Here's how the part is built. I have some questions about the finished solid (model axes, mm). Face numbers are marked on the shaded views. Coordinates: 2 decimals unless noted, no trailing zeros. Write each loop counter-clockwise with the first axis right and the second up, starting at its lowest first coordinate (ties: lowest second). Pieces come first, ordered by that corner, then holes. Notation, with made-up numbers: (30.25, 41.5) -> (38.25, 41.5) arc R16 cw to (38.25, 61.5) -> close; hole circle Ø8 at (-4, 62). An arc over 180 degrees is marked (long way). Put each result on its own line as item: value. Start each with the question number.
Item 1: I want a section at D-D, the plane y = 1.5. State how many separate pieces and enclosed holes the cut face has, then the cut area to 3 significant figures.
Item 2: I want a section at A-A, the plane x = -2.5. List the corners of the cut face in (y, z) for me, then the cut area to 3 significant figures.
Item 3: I want a section at B-B, the plane z = 2.5. List the corners of the cut face in (x, y) for me, then the cut area to 3 significant figures.
Item 4: I want a section at C-C, the plane x = -19.5. List the corners of the cut face in (y, z) for me, then the cut area to 3 significant figures.
Item 5: I need wall thicknesses on line 1 (X direction, y = 0.8, z = 15.66); line 2 (Z direction, x = 25.3, y = 0.75); line 3 (X direction, y = 1.45, z = -8.5). Which ranges of each line are inside material? Lowest first, please. Write a range as [from, to].
Item 6: If we mould it in two halves opening along Y, with no side actions, what happens to the marked faces 1 and 2? For each: released by +Y, released by -Y, zero draft, split by the parting line, or undercut.
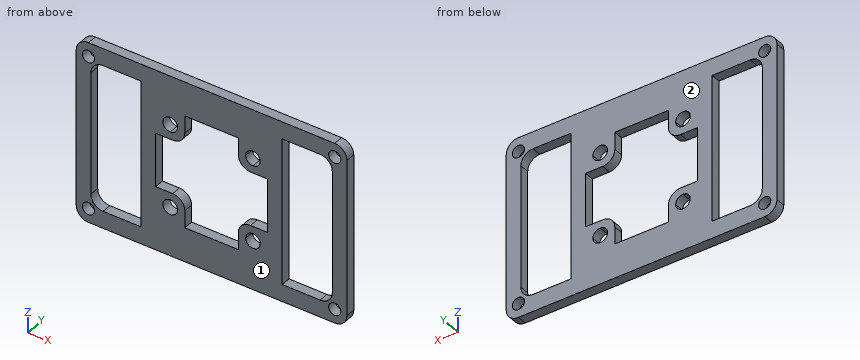
from build123d import *

# Parameters (mm, degrees)
SKETCH1_W           = 55.6
SKETCH1_H           = 37
BOSS_EXTRUDE1_DEPTH = 2
CUT_EXTRUDE2_REACH  = 4
FILLET2_R           = 2.5
CUT_EXTRUDE3_REACH  = 4
CUT_EXTRUDE4_REACH  = 4
SKETCH7_R           = 1.25
CUT_EXTRUDE5_DEPTH  = 10


with BuildPart() as part:
    # Sketch1 → Boss-Extrude1 (new body)
    with BuildSketch(Plane(origin=(0, 0, 0), x_dir=(1, 0, 0), z_dir=(0, 1, 0))):
        Rectangle(SKETCH1_W, SKETCH1_H)
    extrude(amount=BOSS_EXTRUDE1_DEPTH)

    # Sketch5 → Cut-Extrude2 (cut, up to next)
    with BuildSketch(Plane(origin=(0, 2, 0), x_dir=(1, 0, 0), z_dir=(0, 1, 0)), mode=Mode.PRIVATE) as cut_extrude2_sk1:
        with BuildLine():
            Line((5.5, 11.5), (-5.5, 11.5))
            Line((-5.5, 11.5), (-5.5, 8))
            ThreePointArc((-5.5, 8), (-6.232233047, 6.232233047), (-8, 5.5))
            Line((-8, 5.5), (-11.5, 5.5))
            Line((-11.5, 5.5), (-11.5, -5.5))
            Line((-11.5, -5.5), (-8, -5.5))
            ThreePointArc((-8, -5.5), (-6.232233047, -6.232233047), (-5.5, -8))
            Line((-5.5, -8), (-5.5, -11.5))
            Line((-5.5, -11.5), (5.5, -11.5))
            Line((5.5, -11.5), (5.5, -8))
            ThreePointArc((5.5, -8), (6.232233047, -6.232233047), (8, -5.5))
            Line((8, -5.5), (11.5, -5.5))
            Line((11.5, -5.5), (11.5, 5.5))
            Line((11.5, 5.5), (8, 5.5))
            ThreePointArc((8, 5.5), (6.232233047, 6.232233047), (5.5, 8))
            Line((5.5, 8), (5.5, 11.5))
        make_face()
    cut_extrude2_tool1 = extrude(cut_extrude2_sk1.sketch, amount=-CUT_EXTRUDE2_REACH, mode=Mode.PRIVATE) & part.part
    add(cut_extrude2_tool1.solids().sort_by_distance((0, 2, 0))[0], mode=Mode.SUBTRACT)

    # Fillet2
    fillet2_edges = [part.edges().sort_by_distance(p)[0] for p in [
        (27.8, 1, 18.5),
        (-27.8, 1, 18.5),
        (-27.8, 1, -18.5),
        (27.8, 1, -18.5),
    ]]
    fillet(fillet2_edges, radius=FILLET2_R)

    # Sketch6 → Cut-Extrude3 (cut, up to next)
    with BuildSketch(Plane(origin=(0, 2, 0), x_dir=(1, 0, 0), z_dir=(0, 1, 0)), mode=Mode.PRIVATE) as cut_extrude3_sk1:
        with BuildLine():
            Line((-22.3, 15), (-14.5, 15))
            Line((-14.5, 15), (-14.5, -15))
            Line((-14.5, -15), (-22.3, -15))
            ThreePointArc((-22.3, -15), (-24.067766953, -14.267766953), (-24.8, -12.5))
            Line((-24.8, -12.5), (-24.8, 12.5))
            ThreePointArc((-24.8, 12.5), (-24.067766953, 14.267766953), (-22.3, 15))
        make_face()
    cut_extrude3_tool1 = extrude(cut_extrude3_sk1.sketch, amount=-CUT_EXTRUDE3_REACH, mode=Mode.PRIVATE) & part.part
    add(cut_extrude3_tool1.solids().sort_by_distance((-19.60979, 2, 0))[0], mode=Mode.SUBTRACT)
    # Sketch6 → Cut-Extrude3 (cut, up to next)
    with BuildSketch(Plane(origin=(0, 2, 0), x_dir=(1, 0, 0), z_dir=(0, 1, 0)), mode=Mode.PRIVATE) as cut_extrude3_sk2:
        with BuildLine():
            Line((22.3, -15), (14.5, -15))
            Line((14.5, -15), (14.5, 15))
            Line((14.5, 15), (22.3, 15))
            ThreePointArc((22.3, 15), (24.067766953, 14.267766953), (24.8, 12.5))
            Line((24.8, 12.5), (24.8, -12.5))
            ThreePointArc((24.8, -12.5), (24.067766953, -14.267766953), (22.3, -15))
        make_face()
    cut_extrude3_tool2 = extrude(cut_extrude3_sk2.sketch, amount=-CUT_EXTRUDE3_REACH, mode=Mode.PRIVATE) & part.part
    add(cut_extrude3_tool2.solids().sort_by_distance((19.60979, 2, 0))[0], mode=Mode.SUBTRACT)

    # Sketch7 → Cut-Extrude4 (cut, up to next)
    with BuildSketch(Plane(origin=(0, 2, 0), x_dir=(1, 0, 0), z_dir=(0, 1, 0)), mode=Mode.PRIVATE) as cut_extrude4_sk1:
        with Locations((-25.3, 15.66)):
            Circle(SKETCH7_R)
    cut_extrude4_tool1 = extrude(cut_extrude4_sk1.sketch, amount=-CUT_EXTRUDE4_REACH, mode=Mode.PRIVATE) & part.part
    add(cut_extrude4_tool1.solids().sort_by_distance((-25.3, 2, -15.66))[0], mode=Mode.SUBTRACT)
    # Sketch7 → Cut-Extrude4 (cut, up to next)
    with BuildSketch(Plane(origin=(0, 2, 0), x_dir=(1, 0, 0), z_dir=(0, 1, 0)), mode=Mode.PRIVATE) as cut_extrude4_sk2:
        with Locations((25.3, 15.66)):
            Circle(SKETCH7_R)
    cut_extrude4_tool2 = extrude(cut_extrude4_sk2.sketch, amount=-CUT_EXTRUDE4_REACH, mode=Mode.PRIVATE) & part.part
    add(cut_extrude4_tool2.solids().sort_by_distance((25.3, 2, -15.66))[0], mode=Mode.SUBTRACT)
    # Sketch7 → Cut-Extrude4 (cut, up to next)
    with BuildSketch(Plane(origin=(0, 2, 0), x_dir=(1, 0, 0), z_dir=(0, 1, 0)), mode=Mode.PRIVATE) as cut_extrude4_sk3:
        with Locations((25.3, -15.66)):
            Circle(SKETCH7_R)
    cut_extrude4_tool3 = extrude(cut_extrude4_sk3.sketch, amount=-CUT_EXTRUDE4_REACH, mode=Mode.PRIVATE) & part.part
    add(cut_extrude4_tool3.solids().sort_by_distance((25.3, 2, 15.66))[0], mode=Mode.SUBTRACT)
    # Sketch7 → Cut-Extrude4 (cut, up to next)
    with BuildSketch(Plane(origin=(0, 2, 0), x_dir=(1, 0, 0), z_dir=(0, 1, 0)), mode=Mode.PRIVATE) as cut_extrude4_sk4:
        with Locations((-25.3, -15.66)):
            Circle(SKETCH7_R)
    cut_extrude4_tool4 = extrude(cut_extrude4_sk4.sketch, amount=-CUT_EXTRUDE4_REACH, mode=Mode.PRIVATE) & part.part
    add(cut_extrude4_tool4.solids().sort_by_distance((-25.3, 2, 15.66))[0], mode=Mode.SUBTRACT)

    # Sketch3 → Cut-Extrude5 (cut)
    with BuildSketch(Plane(origin=(0, 2, 0), x_dir=(1, 0, 0), z_dir=(0, 1, 0))):
        with BuildLine():
            Line((-8.5, 7), (-8.5, 8.5))
            Line((-8.5, 8.5), (-7, 8.5))
            ThreePointArc((-7, 8.5), (-9.560660172, 9.560660172), (-8.5, 7))
        make_face()
        with BuildLine():
            Line((-7, 8.5), (-8.5, 8.5))
            Line((-8.5, 8.5), (-8.5, 7))
            ThreePointArc((-8.5, 7), (-7.439339828, 7.439339828), (-7, 8.5))
        make_face()
        with BuildLine():
            ThreePointArc((10, 8.5), (8.5, 10), (7, 8.5))
            Line((7, 8.5), (8.5, 8.5))
            Line((8.5, 8.5), (8.5, 7))
            ThreePointArc((8.5, 7), (9.560660172, 7.439339828), (10, 8.5))
        make_face()
        with BuildLine():
            Line((8.5, 8.5), (7, 8.5))
            ThreePointArc((7, 8.5), (7.439339828, 7.439339828), (8.5, 7))
            Line((8.5, 7), (8.5, 8.5))
        make_face()
        with BuildLine():
            ThreePointArc((-7, -8.5), (-7.439339828, -7.439339828), (-8.5, -7))
            Line((-8.5, -7), (-8.5, -8.5))
            Line((-8.5, -8.5), (-7, -8.5))
        make_face()
        with BuildLine():
            Line((-8.5, -8.5), (-8.5, -7))
            ThreePointArc((-8.5, -7), (-9.560660172, -9.560660172), (-7, -8.5))
            Line((-7, -8.5), (-8.5, -8.5))
        make_face()
        with BuildLine():
            ThreePointArc((10, -8.5), (9.560660172, -7.439339828), (8.5, -7))
            Line((8.5, -7), (8.5, -8.5))
            Line((8.5, -8.5), (7, -8.5))
            ThreePointArc((7, -8.5), (8.5, -10), (10, -8.5))
        make_face()
        with BuildLine():
            Line((8.5, -8.5), (8.5, -7))
            ThreePointArc((8.5, -7), (7.439339828, -7.439339828), (7, -8.5))
            Line((7, -8.5), (8.5, -8.5))
        make_face()
    extrude(amount=-CUT_EXTRUDE5_DEPTH, mode=Mode.SUBTRACT)


solid = part.part
Calculated:
1. separate pieces: 1
1. enclosed holes: 11
1. area: 1,000 mm2
2. outline: (0, -18.5) -> (2, -18.5) -> (2, -11.5) -> (0, -11.5) -> close; (0, 11.5) -> (2, 11.5) -> (2, 18.5) -> (0, 18.5) -> close
2. area: 28.0 mm2
3. outline: (-27.8, 0) -> (-24.8, 0) -> (-24.8, 2) -> (-27.8, 2) -> close; (-14.5, 0) -> (-11.5, 0) -> (-11.5, 2) -> (-14.5, 2) -> close; (11.5, 0) -> (14.5, 0) -> (14.5, 2) -> (11.5, 2) -> close; (24.8, 0) -> (27.8, 0) -> (27.8, 2) -> (24.8, 2) -> close
3. area: 24.0 mm2
4. outline: (0, -18.5) -> (2, -18.5) -> (2, -15) -> (0, -15) -> close; (0, 15) -> (2, 15) -> (2, 18.5) -> (0, 18.5) -> close
4. area: 14.0 mm2
5. line 1: x = [-27.8, -26.55], [-24.05, 24.05], [26.55, 27.8]
5. line 2: z = [-18.5, -16.91], [-14.41, 14.41], [16.91, 18.5]
5. line 3: x = [-27.8, -24.8], [-14.5, -10], [-7, -5.5], [5.5, 7], [10, 14.5], [24.8, 27.8]
6. face 1: released by -Y
6. face 2: released by +Y
